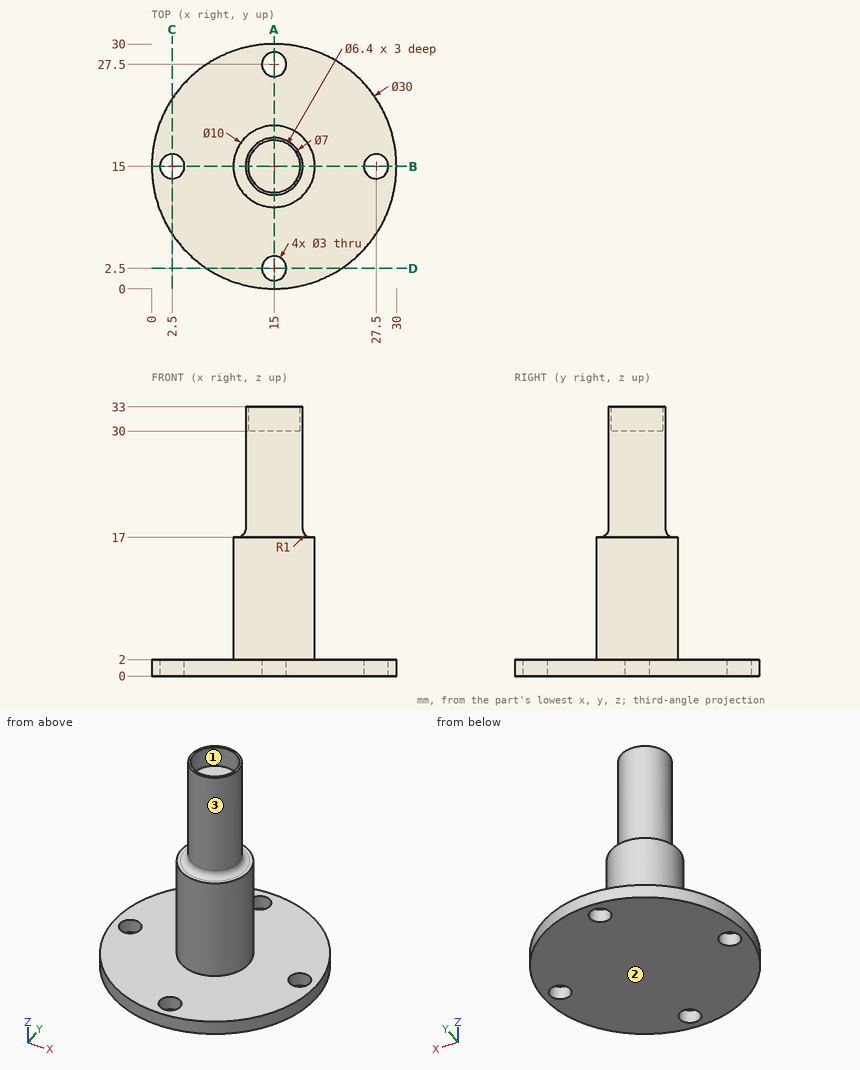
Can you work these out from the drawing? Everything is in mm from the part's minimum corner. Coordinates: 2 decimals unless noted, no trailing zeros. Write each loop counter-clockwise with the first axis right and the second up, starting at its lowest first coordinate (ties: lowest second). Pieces come first, ordered by that corner, then holes. Notation, with made-up numbers: (82, 64.25) -> (131, 64.25) arc R26 ccw to (131, 99.25) -> close; hole circle Ø7 at (82, 29.5). An arc over 180 degrees is marked (long way). Return JSON: item names as keys, results as strings.
(1) We'd pull the mould along X, two halves only. Please class the marked faces 1, 2 and 3: +X half, -X half, draft (parallel to the pull), parting line (faces both ways), or undercut.
Numbers:
{"face 1": "undercut", "face 2": "draft", "face 3": "parting line"}
(2) Imagine slicing it at A-A, the plane x = 15. Please give me the cut outline in (y, z).
Numbers:
{"outline": "(0, 0) -> (1, 0) -> (1, 2) -> (0, 2) -> close; (4, 0) -> (26, 0) -> (26, 2) -> (20, 2) -> (20, 17) -> (19.5, 17) arc R1 cw to (18.5, 18) -> (18.5, 33) -> (18.2, 33) -> (18.2, 30) -> (11.8, 30) -> (11.8, 33) -> (11.5, 33) -> (11.5, 18) arc R1 cw to (10.5, 17) -> (10, 17) -> (10, 2) -> (4, 2) -> close; (29, 0) -> (30, 0) -> (30, 2) -> (29, 2) -> close"}
(3) Imagine slicing it at C-C, the plane x = 2.5. Please give me the cut outline in (y, z), then the cut area to 3 significant figures.
Numbers:
{"outline": "(6.71, 0) -> (13.5, 0) -> (13.5, 2) -> (6.71, 2) -> close; (16.5, 0) -> (23.29, 0) -> (23.29, 2) -> (16.5, 2) -> close", "area": "27.2 mm2"}
(4) I need wall thicknesses on L1, parallel to Y at x = 15, z = 1.45; L2, parallel to Z at x = 5, y = 13; L3, parallel to Y at x = 27.5, z = 1.3. Which ranges of each line are inside material? Lowest first, please.
Numbers:
{"L1": "y = 0 to 1, 4 to 26, 29 to 30", "L2": "z = 0 to 2", "L3": "y = 6.71 to 13.5, 16.5 to 23.29"}
(5) I'm going to push flat-ended pins straight in: pin 1 (15 mm diameter, centred on x = 16, y = 20.5, fed in from +Z); pin 2 (8 mm diameter, centred on x = 25.5, y = 18.5, fed in from +Z); pin 3 (5 mm diameter, centred on x = 15, y = 15, fed in from +Z); pin 4 (5 mm diameter, centred on x = 15.5, z = 17, fed in from +Y). Where does each tip first touch, or does it pass through?
Numbers:
{"pin 1": "stops at z = 33", "pin 2": "stops at z = 2", "pin 3": "stops at z = 30", "pin 4": "stops at y = 20"}
